The model under review builds one solid part; all positions refer to its coordinate system, in mm. A direction names the side the tool comes from. Round coordinates to 2 decimals unless told otherwise and drop trailing zeros. Order: outer loops, then holes, each group sorted by start corner. A loop starts at its lowest first (then second) coordinate and runs counter-clockwise, first axis right, second up. Notation, with made-up numbers: (11.25, -33.75) -> (63.25, -33.75) arc R10 cw to (63.25, -22.75) -> close; hole circle Ø11 at (42.5, -10). An arc over 180 degrees is marked (long way). Use a Markdown table: item, result. Add a question column.
```python
from build123d import *

# Parameters (mm, degrees)
F0_R     = 5.674275
F1_DEPTH = 6.35


with BuildPart() as f1:
    # F0 (on Top) → F1 (new body)
    with BuildSketch(Plane.XY):
        with BuildLine():
            ThreePointArc((29.390265, 10.770578), (22.359371, 27.744657), (5.385291, 34.775551))
            ThreePointArc((5.385291, 34.775551), (-18.619682, 10.770578), (5.385291, -13.234396))
            ThreePointArc((5.385291, -13.234396), (22.359371, -6.203502), (29.390265, 10.770578))
        make_face()
        with Locations((5.385291, 10.770578)):
            Circle(F0_R, mode=Mode.SUBTRACT)
        with BuildLine():
            Line((-16.658982, 48.929192), (-31.542405, 48.929192))
            Line((-31.542405, 48.929192), (-31.542405, -56.622464))
            Line((-31.542405, -56.622464), (-16.658982, -56.622464))
            ThreePointArc((-16.658982, -56.622464), (-12.168854, -54.762592), (-10.308982, -50.272464))
            Line((-10.308982, -50.272464), (-10.308982, -19.584396))
            ThreePointArc((-10.308982, -19.584396), (-8.44911, -15.094267), (-3.958982, -13.234396))
            Line((-3.958982, -13.234396), (5.385291, -13.234396))
            ThreePointArc((5.385291, -13.234396), (-18.619682, 10.770578), (5.385291, 34.775551))
            Line((5.385291, 34.775551), (-3.958982, 34.775551))
            ThreePointArc((-3.958982, 34.775551), (-8.44911, 36.635423), (-10.308982, 41.125551))
            Line((-10.308982, 41.125551), (-10.308982, 42.579192))
            ThreePointArc((-10.308982, 42.579192), (-12.168854, 47.06932), (-16.658982, 48.929192))
        make_face()
    extrude(amount=F1_DEPTH)


solid = f1.part
```
Q1. Insertion check: pin 1 (1 mm diameter, centred on x = -14, z = 3.5, fed in from -Y); pin 2 (3 mm diameter, centred on x = 3, z = 4, fed in from +Y); pin 3 (0.7 mm diameter, centred on y = 42, z = 2.5, fed in from +X). Each pin has a flat end and moves straight along its axis. Give the tip position at first contact, or say it passes through.
Q2. Add section C-C (y = 15). Write out the cut boundary in (x, z), then the cut area to 3 significant figures.
Q3. Add section B-B (x = 8). Write out the cut boundary in (y, z), then the cut area to 3 significant figures.
Q4. Wall thickness on line 1 (X direction, y = -31.5, z = 5); line 2 (X direction, y = 15, z = 2.5); line 3 (Y direction, x = -3, z = 1.5): over which ranges is each line inside the solid? List them lowest first. Write a range as [from, to].
Q5. Add section D-D (y = -26.5). Write out the cut boundary in (x, z).
Q6. Machinability: for faces 1 (the flat face through (-24, 48.929, 3)), 2 (the flat face through (-10.309, -35, 3)), 3 (the flat face through (1, 34.776, 3)), which of the approach directions +Z, -Z, +X, -X, +Y, -Y give a long, thin tool a straight path to every point of the face, cutting with its end or side? Answer none if there is none.
Q7. Add section A-A (z = 4). Write out the cut boundary in (x, y).
Report:
| question | item | result |
|---|---|---|
| 1 | pin 1 | stops at y = -56.24 |
| 1 | pin 2 | stops at y = 34.78 |
| 1 | pin 3 | stops at x = -10.31 |
| 2 | outline | (-31.54, 0) -> (1.6, 0) -> (1.6, 6.35) -> (-31.54, 6.35) -> close; (9.17, 0) -> (29.01, 0) -> (29.01, 6.35) -> (9.17, 6.35) -> close |
| 2 | area | 336 mm² |
| 3 | outline | (-13.09, 0) -> (5.73, 0) -> (5.73, 6.35) -> (-13.09, 6.35) -> close; (15.81, 0) -> (34.63, 0) -> (34.63, 6.35) -> (15.81, 6.35) -> close |
| 3 | area | 239 mm² |
| 4 | line 1 | x = [-31.54, -10.31] |
| 4 | line 2 | x = [-31.54, 1.6], [9.17, 29.01] |
| 4 | line 3 | y = [-13.23, 34.78] |
| 5 | outline | (-31.54, 0) -> (-10.31, 0) -> (-10.31, 6.35) -> (-31.54, 6.35) -> close |
| 6 | face 1 | +Z, -Z, +X, -X, +Y |
| 6 | face 2 | +Z, -Z, +X, -Y |
| 6 | face 3 | +Z, -Z, +X, +Y |
| 7 | outline | (-31.54, -56.62) -> (-16.66, -56.62) arc R6.35 ccw to (-10.31, -50.27) -> (-10.31, -19.58) arc R6.35 cw to (-3.96, -13.23) -> (5.39, -13.23) arc R24 ccw to (5.39, 34.78) -> (-3.96, 34.78) arc R6.35 cw to (-10.31, 41.13) -> (-10.31, 42.58) arc R6.35 ccw to (-16.66, 48.93) -> (-31.54, 48.93) -> close; hole circle Ø11.35 at (5.39, 10.77) |
